Design review of the part built by this model. Coordinates are the model's own, in mm. Face numbers are marked on the shaded views. A direction names the side the tool comes from. Give positions to 0.01 mm unless a question says otherwise; leave off trailing zeros. Write each loop counter-clockwise with the first axis right and the second up, starting at its lowest first coordinate (ties: lowest second). Pieces come first, ordered by that corner, then holes. Notation, with made-up numbers: M -18,41.25 L 2,41.25 A22 ccw 2,73.25 Z; hole C -15.5,78 d9. An arc over 180 degrees is marked long. Write each question's results on one line, items separated by ' | '. Start each with the question number.
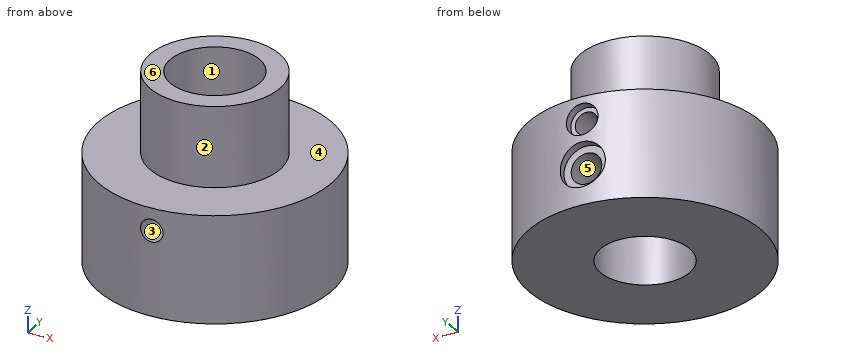
from build123d import *

# Parameters (mm, degrees)
SKETCH2_R                   = 10
CUT_EXTRUDE1_DEPTH          = 56.821142948
CUT_EXTRUDE2_REACH          = 81.821
CUT_EXTRUDE2_END_RADIUS     = 26
CUT_EXTRUDE2_START          = 24
SKETCH3_R                   = 5
SKETCH3_R_2                 = 3.5
M8X1_25_TAPPED_HOLE1_REACH  = 72.285
M8X1_25_TAPPED_HOLE1_BORE_R = 3.4
F_5_0_5_DIAMETER_HOLE1_D    = 5


with BuildPart() as part:
    # Sketch1 → Revolve1 (revolve)
    with BuildSketch(Plane(origin=(0, 0, 0), x_dir=(0, 0, -1), z_dir=(1, 0, 0))):
        Polygon((0, 0), (0, 14.5), (18, 14.5), (18, 26), (42, 26), (42, 0), align=None)
    revolve(axis=Axis((0, 0, -42), (0, 0, 1)))

    # Sketch2 → Cut-Extrude1 (cut, through all)
    with BuildSketch(Plane.XY):
        Circle(SKETCH2_R)
    extrude(amount=-CUT_EXTRUDE1_DEPTH, mode=Mode.SUBTRACT)

    # Cut-Extrude2: up to this cylinder (the profile starts inside it)
    cut_extrude2_end = Plane(origin=(0, 0, -28), z_dir=(0, 0, -1)) * Cylinder(CUT_EXTRUDE2_END_RADIUS, 226.642, mode=Mode.PRIVATE)
    # Sketch3 → Cut-Extrude2 (cut, up to the surface)
    with BuildSketch(Plane(origin=(0, 0, 0), x_dir=(1, 0, 0), z_dir=(0, 1, 0)).offset(CUT_EXTRUDE2_START), mode=Mode.PRIVATE) as cut_extrude2_sk1:
        with Locations(Location((0, 33, 0), (0, 0, 270))):
            Circle(SKETCH3_R)
    cut_extrude2_tool1 = extrude(cut_extrude2_sk1.sketch, amount=CUT_EXTRUDE2_REACH, mode=Mode.PRIVATE) & cut_extrude2_end
    add(cut_extrude2_tool1.solids().sort_by_distance((0, 24, -33))[0], mode=Mode.SUBTRACT)
    # Sketch3 → Cut-Extrude2 (cut, up to the surface)
    with BuildSketch(Plane(origin=(0, 0, 0), x_dir=(1, 0, 0), z_dir=(0, 1, 0)).offset(CUT_EXTRUDE2_START), mode=Mode.PRIVATE) as cut_extrude2_sk2:
        with Locations(Location((0, 23, 0), (0, 0, 270))):
            Circle(SKETCH3_R_2)
    cut_extrude2_tool2 = extrude(cut_extrude2_sk2.sketch, amount=CUT_EXTRUDE2_REACH, mode=Mode.PRIVATE) & cut_extrude2_end
    add(cut_extrude2_tool2.solids().sort_by_distance((0, 24, -23))[0], mode=Mode.SUBTRACT)

    # M8x1.25 Tapped Hole1 bore → M8x1.25 Tapped Hole1 (cut, up to next)
    with BuildSketch(Plane(origin=(0, 24, 0), x_dir=(1, 0, 0), z_dir=(0, 1, 0)), mode=Mode.PRIVATE) as m8x1_25_tapped_hole1_sk1:
        with Locations((0, 33)):
            Circle(M8X1_25_TAPPED_HOLE1_BORE_R)
    m8x1_25_tapped_hole1_tool1 = extrude(m8x1_25_tapped_hole1_sk1.sketch, amount=-M8X1_25_TAPPED_HOLE1_REACH, mode=Mode.PRIVATE) & part.part
    add(m8x1_25_tapped_hole1_tool1.solids().sort_by_distance((0, 24, -33))[0], mode=Mode.SUBTRACT)

    # Ø5.0 (5) Diameter Hole1 (through all)
    with Locations(Plane(origin=(0, 24, 0), x_dir=(1, 0, 0), z_dir=(0, 1, 0))):
        with Locations((0, 23)):
            Hole(F_5_0_5_DIAMETER_HOLE1_D / 2)


solid = part.part
Q1. We need section D-D on y = 18. Write out the cut boundary in (x, z).
Q2. We need section B-B on y = -1.5. Write out the cut boundary in (x, z).
Q3. For the marked faces 4, 5 and 6, list the 3-axis set-ups (+Z, -Z, +X, -X, +Y, -Y) from which the entire face can be reached by the end or side of a thin tool; tool diameter is ignored.
Q4. We need section A-A on x = 0. Count the separate pieces of the cut face and the enclosed holes in it, and give its area (3 significant figures).
Q5. We need section C-C on z = -23. Write out the cut boundary in (x, y), and give its area (3 significant figures).
Q6. Wall thickness on line 1 along Z through (x, y) = (0, 18); line 2 along Z through (x, y) = (0, -15); line 3 along Y through (x, z) = (0, -14): over which ranges is each line inside the solid? List them lowest first. Write a range as from..to.
Q7. For pin 1 Ø12 at (y, z) = (-1.5, -8) entering from -X; pin 2 Ø8 at (y, z) = (-12.5, -31) entering from +X; pin 3 Ø5 at (y, z) = (-6.5, -37.5) entering from -X, all flat-tipped, find the tip position at first contact; note any pin that passes through.
Q8. The part is to be moulded in two halves that separate along Y. For the marked faces 1, 2 and 3, say which applies: pulls with the +Y half, pulls with the -Y half, needs draft (parallel to the pull), parting line crosses it, or undercut.
Answer sheet:
1) outline: M -18.76,-42 L 18.76,-42 L 18.76,-18 L -18.76,-18 Z; hole C 0,-33 d6.8; hole C 0,-23 d5
2) outline: M -25.96,-42 L -9.89,-42 L -9.89,0 L -14.42,0 L -14.42,-18 L -25.96,-18 Z; M 9.89,-42 L 25.96,-42 L 25.96,-18 L 14.42,-18 L 14.42,0 L 9.89,0 Z
3) face 4: +Z | face 5: +Y | face 6: +Z, +X, -X, +Y, -Y
4) separate pieces: 5 | enclosed holes: 0 | area: 651 mm^2
5) outline: M -3.5,24 L -3.5,25.76 A26 ccw -2.5,-25.88 L -2.5,-9.68 A10 cw -2.5,9.68 L -2.5,24 Z; M 2.5,-25.88 A26 ccw 3.5,25.76 L 3.5,24 L 2.5,24 L 2.5,9.68 A10 cw 2.5,-9.68 Z | area: 1,650 mm^2
6) line 1: -42..-36.4, -29.6..-25.5, -20.5..-18 | line 2: -42..-25.5, -20.5..-18 | line 3: -14.5..-10, 10..14.5
7) pin 1: x = -14.5 | pin 2: x = 24.57 | pin 3: x = -25.69
8) face 1: undercut | face 2: parting line crosses it | face 3: needs draft
